```python
from build123d import *

# Parameters (mm, degrees)
SKETCH1_W           = 47
SKETCH1_H           = 47
BOSS_EXTRUDE1_DEPTH = 85
SKETCH2_W           = 47
SKETCH2_H           = 30
CUT_EXTRUDE1_DEPTH  = 20
SKETCH3_W           = 27
SKETCH3_H           = 29.949158553
CUT_EXTRUDE2_DEPTH  = 20
SKETCH4_W           = 27
SKETCH4_H           = 30
CUT_EXTRUDE3_DEPTH  = 20
SKETCH5_W           = 7
SKETCH5_H           = 30
CUT_EXTRUDE4_DEPTH  = 20
SKETCH6_W           = 17.880231582
SKETCH6_H           = 18.920879981
BOSS_EXTRUDE2_DEPTH = 18
SKETCH7_R           = 33
BOSS_EXTRUDE4_DEPTH = 7
SKETCH9_R           = 32.855450218
BOSS_EXTRUDE5_DEPTH = 1


with BuildPart() as part:
    # Sketch1 → Boss-Extrude1 (new body)
    with BuildSketch(Plane(origin=(0, 0, 0), x_dir=(1, 0, 0), z_dir=(0, 1, 0))):
        with Locations((23.5, 23.5)):
            Rectangle(SKETCH1_W, SKETCH1_H)
    extrude(amount=BOSS_EXTRUDE1_DEPTH)

    # Sketch2 → Cut-Extrude1 (cut)
    with BuildSketch(Plane.XY):
        with Locations((23.5, 15)):
            Rectangle(SKETCH2_W, SKETCH2_H)
    extrude(amount=-CUT_EXTRUDE1_DEPTH, mode=Mode.SUBTRACT)

    # Sketch3 → Cut-Extrude2 (cut)
    with BuildSketch(Plane.ZY):
        with Locations((-33.5, 14.974579277)):
            Rectangle(SKETCH3_W, SKETCH3_H)
    extrude(amount=-CUT_EXTRUDE2_DEPTH, mode=Mode.SUBTRACT)

    # Sketch4 → Cut-Extrude3 (cut)
    with BuildSketch(Plane(origin=(0, 0, -47), x_dir=(-1, 0, 0), z_dir=(0, 0, -1))):
        with Locations((-33.5, 15)):
            Rectangle(SKETCH4_W, SKETCH4_H)
    extrude(amount=-CUT_EXTRUDE3_DEPTH, mode=Mode.SUBTRACT)

    # Sketch5 → Cut-Extrude4 (cut)
    with BuildSketch(Plane(origin=(47, 0, 0), x_dir=(0, 0, -1), z_dir=(1, 0, 0))):
        with Locations((23.5, 15)):
            Rectangle(SKETCH5_W, SKETCH5_H)
    extrude(amount=-CUT_EXTRUDE4_DEPTH, mode=Mode.SUBTRACT)

    # Sketch6 → Boss-Extrude2 (add)
    with BuildSketch(Plane(origin=(0, 85, 0), x_dir=(1, 0, 0), z_dir=(0, 1, 0))):
        with Locations((24.162230799, 21.773469702)):
            Rectangle(SKETCH6_W, SKETCH6_H)
    extrude(amount=BOSS_EXTRUDE2_DEPTH)

    # Sketch7 → Boss-Extrude4 (add)
    with BuildSketch(Plane(origin=(0, 103, 0), x_dir=(1, 0, 0), z_dir=(0, 1, 0))):
        with Locations((23.29896565, 23.29896565)):
            Circle(SKETCH7_R)
    extrude(amount=BOSS_EXTRUDE4_DEPTH)

    # Sketch9 → Boss-Extrude5 (add)
    with BuildSketch(Plane.XZ):
        with Locations((22.961502761, -23.5)):
            Circle(SKETCH9_R)
    extrude(amount=BOSS_EXTRUDE5_DEPTH)


solid = part.part
```
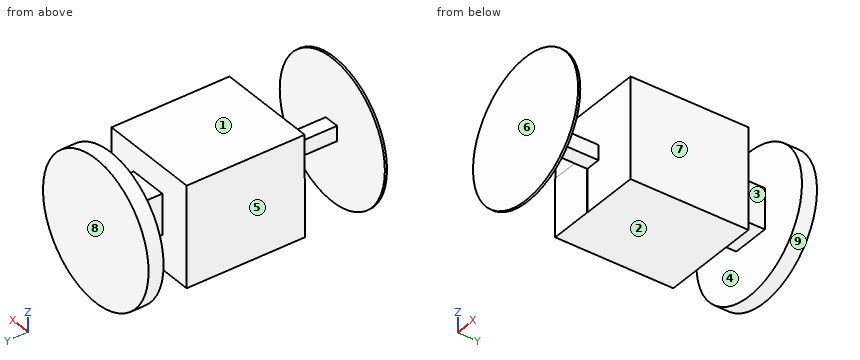
The model under review builds one solid part; all positions refer to its coordinate system, in mm. Face numbers are marked on the shaded views. A direction names the side the tool comes from. Give positions to 0.01 mm unless a question says otherwise; leave off trailing zeros. Write each loop counter-clockwise with the first axis right and the second up, starting at its lowest first coordinate (ties: lowest second). Pieces come first, ordered by that corner, then holes. Notation, with made-up numbers: M -26.75,-22 L -14.75,-22 A9 cw -14.75,-5 Z; hole C 10,87.25 d3. An arc over 180 degrees is marked long. Answer in a Markdown table with one row per item.
Item 1: For P1, Ø5.5, axis at y = 94, z = -20.5, coming from the -X side; P2, Ø1.5, axis at x = 2, y = 63, coming from the -Z side; P3, Ø7.5, axis at x = 23.5, y = 20.5, coming from the -Z side, all flat-tipped, find the tip position at first contact; note any pin that passes through.
Check sheet entries:
| item | result |
|---|---|
| P1 | x = 15.22 |
| P2 | z = -47 |
| P3 | z = -27 |
Item 2: Tool access review of the marked faces 1, 2, 3, 4 and 5: name each direction out of +Z, -Z, +X, -X, +Y, -Y from which nothing blocks a thin tool from reaching the whole face with its end or side.
Check sheet entries:
| item | result |
|---|---|
| face 1 | +Z, +X, -X |
| face 2 | -Z, +X, -X |
| face 3 | +Z, -Z, +X |
| face 4 | none |
| face 5 | +Z, -Z, -X |
Item 3: For line 1 along Y through (x, z) = (46, -10); line 2 along Y through (x, z) = (2, -22); line 3 along Y through (x, z) = (27, -50.5), list the stretches that pass through material, from the lowest coordinate up.
Check sheet entries:
| item | result |
|---|---|
| line 1 | -1 to 0, 30 to 85, 103 to 110 |
| line 2 | -1 to 0, 29.95 to 85, 103 to 110 |
| line 3 | -1 to 0, 103 to 110 |
Item 4: Add section D-D on z = -30. Give the boundary of the cut face in (x, y), plus the area to 3 significant figures.
Check sheet entries:
| item | result |
|---|---|
| outline | M -9.24,-1 L 55.17,-1 L 55.17,0 L -9.24,0 Z; M -9.01,103 L 15.22,103 L 15.22,85 L 0,85 L 0,29.95 L 20,29.95 L 20,30 L 47,30 L 47,85 L 33.1,85 L 33.1,103 L 55.61,103 L 55.61,110 L -9.01,110 Z |
| area | 3,420 mm2 |
Item 5: Draft analysis for pull direction Y (two halves, no side actions). For the marked faces 6, 7, 8 and 9, state which applies: +Y half, -Y half, draft (parallel to the pull), parting line (faces both ways), or undercut.
Check sheet entries:
| item | result |
|---|---|
| face 6 | -Y half |
| face 7 | undercut |
| face 8 | +Y half |
| face 9 | draft |
Item 6: Add section A-A on x = 39. Give the boundary of the cut face in (y, z), plus the area to 3 significant figures.
Check sheet entries:
| item | result |
|---|---|
| outline | M -1,-52.17 L 0,-52.17 L 0,5.17 L -1,5.17 Z; M 30,-47 L 85,-47 L 85,0 L 30,0 Z; M 103,-52.32 L 110,-52.32 L 110,5.73 L 103,5.73 Z |
| area | 3,050 mm2 |
Item 7: Add section C-C on z = -8. Give the boundary of the cut face in (x, y).
Check sheet entries:
| item | result |
|---|---|
| outline | M -6.01,-1 L 51.93,-1 L 51.93,0 L -6.01,0 Z; M -5.94,103 L 52.54,103 L 52.54,110 L -5.94,110 Z; M 0,30 L 47,30 L 47,85 L 0,85 Z |
Item 8: Add section B-B on x = 31.5. Give the boundary of the cut face in (y, z), plus the area to 3 significant figures.
Check sheet entries:
| item | result |
|---|---|
| outline | M -1,-55.23 L 0,-55.23 L 0,8.23 L -1,8.23 Z; M 30,-47 L 85,-47 L 85,-31.23 L 103,-31.23 L 103,-55.26 L 110,-55.26 L 110,8.67 L 103,8.67 L 103,-12.31 L 85,-12.31 L 85,0 L 30,0 Z |
| area | 3,440 mm2 |
